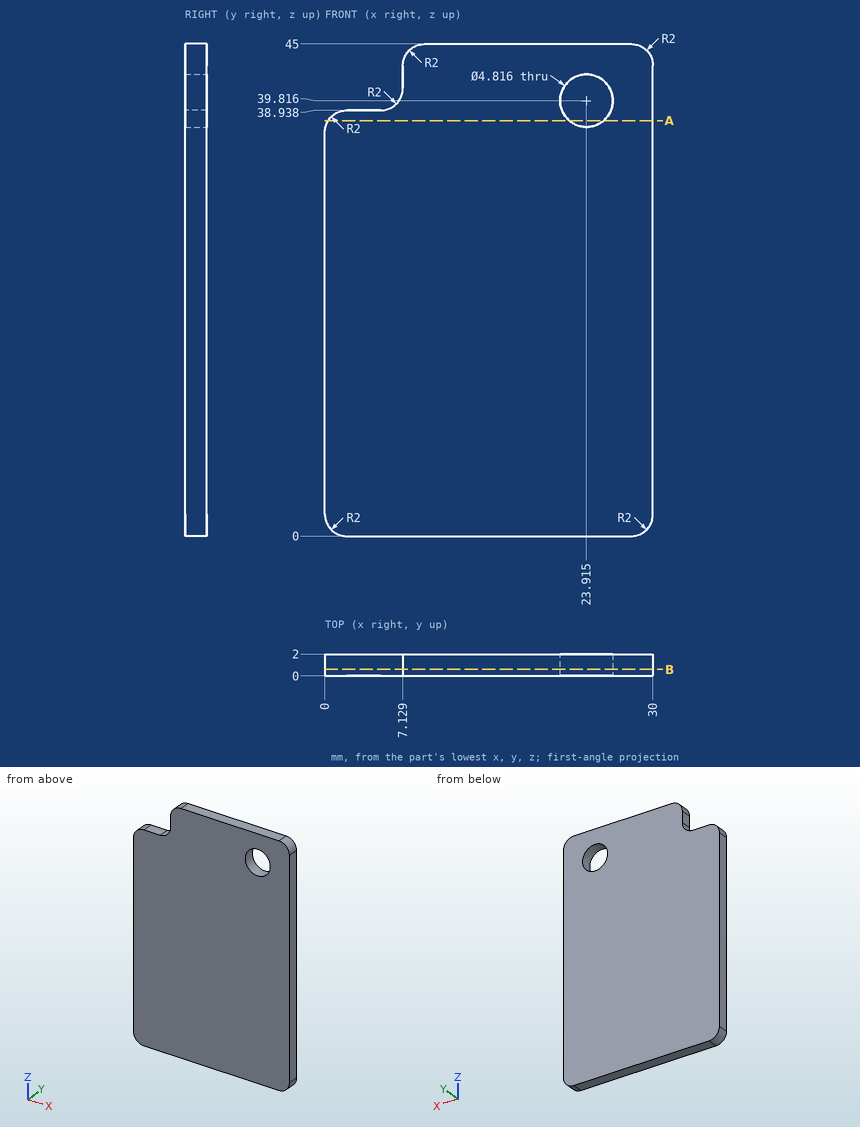
Drawing for the job (mm, zero at the part's lowest x, y, z). Coordinates: 2 decimals unless noted, no trailing zeros. Order: outer loops, then holes, each group sorted by start corner. A loop starts at its lowest first (then second) coordinate and runs counter-clockwise, first axis right, second up. Notation, with made-up numbers: (27.25, 10) -> (68.25, 10) arc R23 cw to (68.25, 32) -> close; hole circle Ø6 at (45.5, 2). An arc over 180 degrees is marked (long way). One line per item, written item: value.
(1) Slice it at A-A, the plane z = 38. List the corners of the cut face in (x, y) (1 decimal).
Checked values:
outline: (0.3, 0) -> (22.3, 0) -> (22.3, 2) -> (0.3, 2) -> close; (25.5, 0) -> (30, 0) -> (30, 2) -> (25.5, 2) -> close
(2) Drop a flat-ended pin along its axis: pin 1 Ø1 at (x, y) = (4, 1.5) entering from +Z. Give the stop position or say it passes through.
Checked values:
pin 1: z = 38.94
(3) Probe line 1 (X direction, y = 0.8, z = 38) (1 decimal); line 2 (Z direction, x = 7.5, y = 1.25). List the from-to ranges inside material, lowest first. Write a range as [from, to].
Checked values:
line 1: [0.3, 22.3], [25.5, 30]
line 2: [0, 44.16]
(4) Slice it at B-B, the plane y = 0.6. List the corners of the cut face in (x, z) (1 decimal).
Checked values:
outline: (0, 2) arc R2 ccw to (2, 0) -> (28, 0) arc R2 ccw to (30, 2) -> (30, 43) arc R2 ccw to (28, 45) -> (9.1, 45) arc R2 ccw to (7.1, 43) -> (7.1, 40.9) arc R2 cw to (5.1, 38.9) -> (2, 38.9) arc R2 ccw to (0, 36.9) -> close; hole circle Ø4.8 at (23.9, 39.8)
